Check sheet for the modelled part. Datum: model origin and axes. Units: mm. A direction names the side the tool comes from. Round coordinates to 2 decimals unless told otherwise and drop trailing zeros. Write each loop counter-clockwise with the first axis right and the second up, starting at its lowest first coordinate (ties: lowest second). Pieces come first, ordered by that corner, then holes. Notation, with made-up numbers: (81, 16.25) -> (105, 16.25) arc R14 cw to (105, 35.25) -> close; hole circle Ø7 at (21.25, 35.25). An arc over 180 degrees is marked (long way). One line per item, written item: value.
Autodesk Inventor part; units mm, degrees
ref_plane "YZ Plane" through (0, 0, 0) normal (1, 0, 0) x (0, 1, 0)
ref_plane "XZ Plane" through (0, 0, 0) normal (0, 1, 0) x (-1, 0, 0)
ref_plane "XY Plane" through (0, 0, 0) normal (0, 0, 1) x (1, 0, 0)
sketch "Sketch6" plane through (0, 0, 0) normal (1, 0, 0) x (0, 1, 0)
  point P0 (0, 0)
sketch "Sketch7" plane through (0, 0, 0) normal (1, 0, 0) x (0, 1, 0)
  line L0 (-2.5, -13.1614) -> (2.5, -13.1614)
  line L1 (2.5, 12.8386) -> (-2.5, 12.8386)
  circle A0 centre (0, 0) radius 0.9858
  line L2 (9, 1.55) -> (9, -1.55)
  line L3 (-9, -1.55) -> (-9, 1.55)
  line L4 (2.5, 1.55) -> (9, 1.55)
  line L5 (-9, 1.55) -> (-2.5, 1.55)
  line L6 (-2.5, -1.55) -> (-9, -1.55)
  line L7 (9, -1.55) -> (2.5, -1.55)
  line L8 (2.5, 1.55) -> (2.5, 12.8386)
  line L9 (2.5, -13.1614) -> (2.5, -1.55)
  line L10 (-2.5, -1.55) -> (-2.5, -13.1614)
  line L11 (-2.5, 12.8386) -> (-2.5, 1.55)
  point P0 (-9, 0)
  point P1 (0, 12.8386)
  point P2 (9, 0)
  point P3 (0, -13.1614)
  dimension "d85" = 5
  dimension "d86" = 3.1
  dimension "d90" = 26
  dimension "d91" = 3.1
  dimension "d92" = 5
  dimension "d93" = 18
extrude "Extrusion3" add sketch "Sketch7" along normal blind 3
fillet "Fillet1" radius 1 1 edges at (1.5, 9, 1.55)
fillet "Fillet2" radius 1 1 edges at (1.5, 9, -1.55)
fillet "Fillet3" radius 1 1 edges at (1.5, -9, -1.55)
fillet "Fillet4" radius 1 1 edges at (1.5, -9, 1.55)
fillet "Fillet5" radius 2 1 edges at (1.5, -2.5, 12.8386)
fillet "Fillet6" radius 2 1 edges at (1.5, 2.5, 12.8386)
fillet "Fillet7" radius 2 1 edges at (1.5, 2.5, -13.1614)
fillet "Fillet8" radius 2 1 edges at (1.5, -2.5, -13.1614)
properties part number "6P-016 cutout"
Item 1: Thickness scan on line 1 (Z direction, x = 1.65, y = 0); line 2 (Y direction, x = 1.8, z = 7.5); line 3 (Z direction, x = 2.8, y = -6.5). Record the ranges inside material, lowest first.
Answer:
line 1: z = -13.16 to -0.99, 0.99 to 12.84
line 2: y = -2.5 to 2.5
line 3: z = -1.55 to 1.55
Item 2: Sectioned sample at A-A on y = 0. Enter the section's corners in (x, z).
Answer:
outline: (0, -13.16) -> (3, -13.16) -> (3, -0.99) -> (0, -0.99) -> close; (0, 0.99) -> (3, 0.99) -> (3, 12.84) -> (0, 12.84) -> close
Item 3: Depth check by flat-ended pin: P1, Ø1.5, axis at x = 1.5, y = 4.5, coming from the +Z side; P2, Ø0.9, axis at x = 1.5, z = 5.5, coming from the +Y side; P3, Ø1.5, axis at x = 2, y = -4.5, coming from the -Z side. Enter the tip coordinate at first touch or a pass-through.
Answer:
P1: stops at z = 1.55
P2: stops at y = 2.5
P3: stops at z = -1.55
Item 4: Sectioned sample at D-D on y = 3.75. Enter the section's corners in (x, z).
Answer:
outline: (0, -1.55) -> (3, -1.55) -> (3, 1.55) -> (0, 1.55) -> close
Item 5: Sectioned sample at B-B on z = 0. Enter the section's corners in (x, y), and give its area (3 significant figures).
Answer:
outline: (0, -9) -> (3, -9) -> (3, -0.99) -> (0, -0.99) -> close; (0, 0.99) -> (3, 0.99) -> (3, 9) -> (0, 9) -> close
area: 48.1 mm^2
Item 6: Sectioned sample at C-C on x = 1.9. Enter the section's corners in (y, z).
Answer:
outline: (-9, -0.55) arc R1 ccw to (-8, -1.55) -> (-2.5, -1.55) -> (-2.5, -11.16) arc R2 ccw to (-0.5, -13.16) -> (0.5, -13.16) arc R2 ccw to (2.5, -11.16) -> (2.5, -1.55) -> (8, -1.55) arc R1 ccw to (9, -0.55) -> (9, 0.55) arc R1 ccw to (8, 1.55) -> (2.5, 1.55) -> (2.5, 10.84) arc R2 ccw to (0.5, 12.84) -> (-0.5, 12.84) arc R2 ccw to (-2.5, 10.84) -> (-2.5, 1.55) -> (-8, 1.55) arc R1 ccw to (-9, 0.55) -> close; hole circle Ø1.97 at (0, 0)
Item 7: Tool access check on faces 1 (the flat face through (1, 2.5, -6)), 2 (the flat face through (1, 5, 1.55)), 3 (the flat face through (1, -2.5, -6)), 4 (the flat face through (1, -2.5, 6)). Record the directions out of +Z, -Z, +X, -X, +Y, -Y that give a thin tool (end or side, any length) a straight path to the whole face; none if there is none.
Answer:
face 1: -Z, +X, -X, +Y
face 2: +Z, +X, -X, +Y
face 3: -Z, +X, -X, -Y
face 4: +Z, +X, -X, -Y
